Source: CAD feature listing. Evaluate the final solid. Frame: model axes, mm. A direction names the side the tool comes from. Give positions to 0.01 mm unless a question says otherwise; leave off trailing zeros. Order: outer loops, then holes, each group sorted by start corner. A loop starts at its lowest first (then second) coordinate and runs counter-clockwise, first axis right, second up.
Autodesk Inventor part; units mm, degrees
ref_plane "Work Plane1" through (0, 38.2, 0) normal (0, -1, 0) x (1, 0, 0)
ref_plane "YZ Plane" through (0, 0, 0) normal (1, 0, 0) x (0, 1, 0)
ref_plane "XZ Plane" through (0, 0, 0) normal (0, 1, 0) x (-1, 0, 0)
sketch "Sketch1" plane through (0, 0, 0) normal (0, 1, 0) x (-1, 0, 0)
  circle A0 centre (0, 0) radius 1.15
  circle A1 centre (0, 0) radius 2
  line L0 (-2, 2) -> (2, 2)
  line L1 (2, 2) -> (2, -2)
  line L2 (2, -2) -> (-2, -2)
  line L3 (-2, -2) -> (-2, 2)
  line L4 (-2, 2) -> (2, -2) construction
  line L5 (2, 2) -> (-2, -2) construction
  dimension "d0" = 2.3
  dimension "d1" = 4
extrude "Extrusion1" add sketch "Sketch1" along normal blind 5
sketch "Sketch2" plane through (0, 5, 0) normal (0, 1, 0) x (1, 0, 0)
  line L0 (2, 2) -> (-2, 2)
  line L1 (-2, 2) -> (-2, -2)
  line L2 (-2, -2) -> (2, -2)
  line L3 (2, -2) -> (2, 2)
  circle A0 centre (0, 0) radius 1.15
extrude "Extrusion2" add sketch "Sketch2" along normal blind 3 contours L3 L2 L1 L0 | A0
sketch "Sketch3" plane through (0, 8, 0) normal (0, 1, 0) x (1, 0, 0)
  line L0 (1.5, -1.5) -> (-1.5, -1.5)
  line L1 (-1.5, -1.5) -> (-1.5, 1.5)
  line L2 (-1.5, 1.5) -> (1.5, 1.5)
  line L3 (1.5, 1.5) -> (1.5, -1.5)
  line L4 (1.5, -1.5) -> (-1.5, 1.5) construction
  line L5 (-1.5, -1.5) -> (1.5, 1.5) construction
  point P0 (0, 0)
  dimension "d6" = 3
extrude "Extrusion3" add sketch "Sketch3" along normal blind 44.25
ref_plane "Work Plane1" through (0, 38.2, 0) normal (0, -1, 0) x (1, 0, 0)
mirror "Mirror1" about plane through (0, 38.2, 0) normal (0, -1, 0) of "Extrusion3", "Extrusion1", "Extrusion2"
properties part number "clamshell cross link" material "ABS Plastic"
1) Pull-direction query (X, two-part tool) for faces 1 (the face through (2, 4, 0)), 2 (the face through (-1.7, 68.4, 0)), 3 (the face through (0.91, 73.94, -0.7)); classes: +X half, -X half, draft (parallel to the pull), parting line (faces both ways), or undercut.
Checks:
face 1: +X half
face 2: draft
face 3: undercut
2) Ray query, L1, parallel to Z at x = 0, y = 73.15; L2, parallel to Y at x = -1.6, z = 0.5; L3, parallel to Z at x = -0.3, y = 9. Return the intervals inside material, ascending.
Checks:
L1: z = -2 to -1.15, 1.15 to 2
L2: y = 0 to 8, 68.4 to 76.4
L3: z = -1.5 to 1.5
3) Reachability of faces 4 (the face through (1.5, 39, 0)), 5 (the face through (0.91, 2.46, 0.7)), 6 (the face through (0, 39, -1.5)) from +Z, -Z, +X, -X, +Y, -Y: full face, straight path, thin tool, end or side. Return the list, or none.
Checks:
face 4: +Z, -Z, +X
face 5: -Y
face 6: -Z, +X, -X
4) First-contact query: pin 1 Ø2 at (y, z) = (20, -1) entering from +X; pin 2 Ø1.4 at (x, z) = (0, 0) entering from +Y; pin 3 Ø1.5 at (y, z) = (36, 0) entering from -X. Flat tips, straight axial feed; report the tip coordinate or a pass-through.
Checks:
pin 1: stops at x = 1.5
pin 2: stops at y = 71.4
pin 3: stops at x = -1.5
5) Section query B-B on z = 0. Output: boundary loops of the cut face in (x, y), and give its area (3 significant figures).
Checks:
outline: (-2, 0) - (-1.15, 0) - (-1.15, 5) - (1.15, 5) - (1.15, 0) - (2, 0) - (2, 8) - (1.5, 8) - (1.5, 68.4) - (2, 68.4) - (2, 76.4) - (1.15, 76.4) - (1.15, 71.4) - (-1.15, 71.4) - (-1.15, 76.4) - (-2, 76.4) - (-2, 68.4) - (-1.5, 68.4) - (-1.5, 8) - (-2, 8) - close
area: 222 mm2
6) Section query C-C on y = 50.5. Output: boundary loops of the cut face in (x, z).
Checks:
outline: (-1.5, -1.5) - (1.5, -1.5) - (1.5, 1.5) - (-1.5, 1.5) - close
7) Section query A-A on x = 0. Output: boundary loops of the cut face in (y, z).
Checks:
outline: (0, -2) - (8, -2) - (8, -1.5) - (68.4, -1.5) - (68.4, -2) - (76.4, -2) - (76.4, -1.15) - (71.4, -1.15) - (71.4, 1.15) - (76.4, 1.15) - (76.4, 2) - (68.4, 2) - (68.4, 1.5) - (8, 1.5) - (8, 2) - (0, 2) - (0, 1.15) - (5, 1.15) - (5, -1.15) - (0, -1.15) - close
